Design review of the part built by this model. Coordinates are the model's own, in mm. Give positions to 0.01 mm unless a question says otherwise; leave off trailing zeros. Loops run counter-clockwise (first coordinate to the right, second up) from the corner with the lowest first, then second, coordinate; pieces in that order, holes last. Notation, with made-up numbers: M -7,-27 L 51,-27 A30 cw 51,9 Z; hole C 16,11 d5. An arc over 180 degrees is marked long. Use CSV: the item, a comma, the result in double quotes.
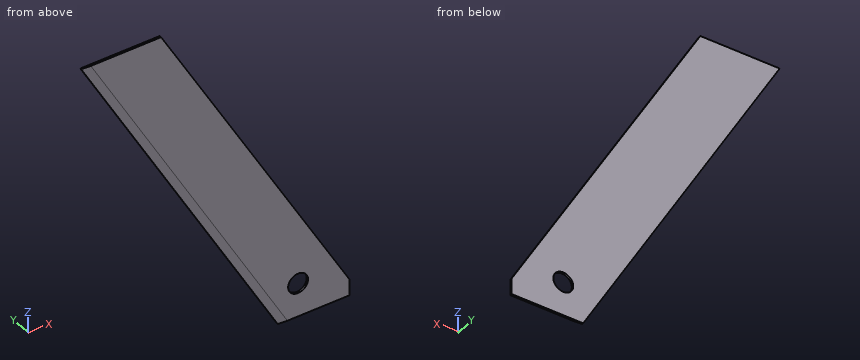
from build123d import *

# Parameters (mm, degrees)
SKETCH_R      = 2.5
PAD_DEPTH     = 0.5
CHAMFER_SIZE2 = 2
CHAMFER_SIZE  = 0.2


with BuildPart() as part:
    # Sketch → Pad (new body)
    with BuildSketch(Plane.XZ):
        Polygon((0, 0), (18, 0), (18, 4), (-29.5, 86.272413), (-49.5, 86.272413), align=None)
        with Locations((5, 8.5)):
            Circle(SKETCH_R, mode=Mode.SUBTRACT)
    extrude(amount=PAD_DEPTH)

    # Chamfer
    chamfer_edges = [part.edges().sort_by_distance(p)[0] for p in [
        (-24.75, -0.5, 43.136207),
    ]]
    chamfer_side = part.faces().sort_by_distance((-24.75, -0.25, 43.136207))[0]
    chamfer(chamfer_edges, length=CHAMFER_SIZE, length2=CHAMFER_SIZE2, reference=chamfer_side)


solid = part.part
(1) We need section B-B on x = 5. State the section outline as (y, z) points.
A:
outline,"M -0.5,0 L 0,0 L 0,6 L -0.5,6 Z; M -0.5,11 L 0,11 L 0,26.52 L -0.5,26.52 Z"
(2) We need section C-C on z = 8.5. State the section outline as (x, y) points.
A:
outline,"M -4.88,-0.3 L -2.57,-0.5 L 2.5,-0.5 L 2.5,0 L -4.88,0 Z; M 7.5,-0.5 L 15.4,-0.5 L 15.4,0 L 7.5,0 Z"
(3) Wall thickness on line 1 along Z through (x, y) = (5, -0.4); line 2 along X through (y, z) = (-0.2, 43.5); line 3 along X through (y, z) = (-0.1, 9.5): over which ranges is each line inside the solid? List them lowest first. Write a range as [from, to].
A:
line 1,"[0, 6], [11, 26.52]"
line 2,"[-24.96, -4.81]"
line 3,"[-5.45, 2.71], [7.29, 14.82]"
(4) We need section A-A on y = -0.1. State the section outline as (x, z) points.
A:
outline,"M -49.5,86.27 L 0,0 L 18,0 L 18,4 L -29.5,86.27 Z; hole C 5,8.5 d5"
(5) We need section D-D on z = 31.5. State the section outline as (x, y) points.
A:
outline,"M -18.07,-0.3 L -15.77,-0.5 L 2.12,-0.5 L 2.12,0 L -18.07,0 Z"
